```python
from build123d import *

# Parameters (mm, degrees)
F4_W = 5
F4_H = 100
F6_R = 20
F7_R = 40


with BuildPart() as f5:
    # F5: sweep along a path in F0, F2
    with BuildLine(Plane.XZ) as f5_path:
        Line((0, -150), (0, 0))
        Line((0, 0), (300, 0))
    with BuildLine(Plane.YZ.offset(300)) as f5_path_2:
        Line((0, 0), (300, 0))
        Line((300, 0), (475, 303.1088913246))
    # F4 (on plane+point) → F5 (sweep)
    with BuildSketch(Plane.XY.offset(-150)):
        Rectangle(F4_W, F4_H)
    sweep(path=f5_path.line + f5_path_2.line, transition=Transition.RIGHT)

    # F6
    f6_edges = [f5.edges().sort_by_distance(p)[0] for p in [
        (2.5, 0, -2.5),
        (300, 298.556624, 2.5),
        (300, 301.443376, -2.5),
    ]]
    fillet(f6_edges, radius=F6_R)

    # F7
    f7_edges = [f5.edges().sort_by_distance(p)[0] for p in [
        (350, -50, 0),
        (250, 50, 0),
        (350, 475, 303.108891),
        (250, 475, 303.108891),
        (0, -50, -150),
        (0, 50, -150),
    ]]
    fillet(f7_edges, radius=F7_R)


solid = f5.part
```
Input: part model. Units: mm. Frame: model coordinates. A direction names the side the tool comes from. Coordinates: 2 decimals unless noted, no trailing zeros. Order: outer loops, then holes, each group sorted by start corner. A loop starts at its lowest first (then second) coordinate and runs counter-clockwise, first axis right, second up. Notation, with made-up numbers: (67, 55) - (125, 55) arc R25 cw to (125, 92) - close; hole circle Ø5 at (5.25, 1.5). An arc over 180 degrees is marked (long way). Return JSON: item names as keys, results as strings.
Q1. Access query for faces 1 (the flat face through (261, 80, -2.5)), 2 (the flat face through (130, -50, 1)), 3 (the flat face through (215, 46, 2.5)), 4 (the flat face through (57, 50, 1)). Directions: +Z, -Z, +X, -X, +Y, -Y. A direction counts if a zero-diameter tool reaches every point of the face in a straight line with its end or side. Return the directions, or none.
The answers:
{"face 1": "-Z, +X, +Y, -Y", "face 2": "+Z, -Z, +X, -X, -Y", "face 3": "+Z, +X, -X, -Y", "face 4": "+Z, -Z, -X, +Y"}
Q2. Ray query, probe 1 along Z at (x, y) = (283.5, 114); probe 2 along Y at (x, z) = (254, 121); probe 3 along Z at (x, y) = (290, 337). Return the intervals inside material, ascending.
The answers:
{"probe 1": "z = -2.5 to 2.5", "probe 2": "y = 366.97 to 372.75", "probe 3": "z = 59.09 to 69.09"}
Q3. First-contact query: pin 1 (12 mm diameter, centred on x = 268, y = 260.5, fed in from +Z). Flat tip, straight axial feed; report the tip coordinate or a pass-through.
The answers:
{"pin 1": "stops at z = 2.5"}
Q4. Cut plane A-A (y = -1). Return loops of the section in (x, z), then the cut area to 3 significant figures.
The answers:
{"outline": "(-2.5, -150) - (2.5, -150) - (2.5, -22.5) arc R20 cw to (22.5, -2.5) - (350, -2.5) - (350, 2.5) - (-2.5, 2.5) - close", "area": "2,590 mm2"}
Q5. Cut plane C-C (z = -65). Return loops of the section in (x, y), then the cut area to 3 significant figures.
The answers:
{"outline": "(-2.5, -50) - (2.5, -50) - (2.5, 50) - (-2.5, 50) - close", "area": "500 mm2"}
Q6. Cut plane D-D (x = 128). Return loops of the section in (y, z), then the cut area to 3 significant figures.
The answers:
{"outline": "(-50, -2.5) - (50, -2.5) - (50, 2.5) - (-50, 2.5) - close", "area": "500 mm2"}
Q7. Cut plane B-B (x = 329.5). Return loops of the section in (y, z).
The answers:
{"outline": "(-44.92, -2.5) - (289.9, -2.5) arc R20 ccw to (307.22, 7.5) - (474.63, 297.46) - (470.3, 299.96) - (304.33, 12.5) arc R20 cw to (287.01, 2.5) - (-44.92, 2.5) - close"}
